Autodesk Inventor part; units mm, degrees
ref_plane "YZ Plane" through (0, 0, 0) normal (1, 0, 0) x (0, 1, 0)
ref_plane "XZ Plane" through (0, 0, 0) normal (0, 1, 0) x (-1, 0, 0)
ref_plane "XY Plane" through (0, 0, 0) normal (0, 0, 1) x (1, 0, 0)
sketch "Sketch1" plane through (0, 0, 0) normal (0, 0, 1) x (1, 0, 0)
  line L0 (0, 0) -> (10, 0)
  line L1 (10, 0) -> (10, 6)
  line L2 (10, 6) -> (0, 6)
  line L3 (0, 6) -> (0, 0)
  dimension "d0" = 10
  dimension "d1" = 6
extrude "Extrusion1" add sketch "Sketch1" along normal blind 4
sketch "Sketch2" plane through (0, 0, 4) normal (0, 0, 1) x (1, 0, 0)
  line L0 (1, 1) -> (9, 1)
  line L1 (9, 1) -> (9, 5)
  line L2 (9, 5) -> (1, 5)
  line L3 (1, 5) -> (1, 1)
  point P0 (0, 0)
  dimension "d4" = 8
  dimension "d5" = 4
extrude "Extrusion2" cut sketch "Sketch2" against normal blind 2.5
sketch "Sketch5" plane through (1, 1, 4) normal (0, 1, 0) x (1, 0, 0)
  circle A0 centre (1, 0.5) radius 0.25
  point P0 (-1, 4)
  dimension "d14" = 0.5
sketch "Sketch6" plane through (1, 1, 4) normal (0, 1, 0) x (1, 0, 0)
  circle A0 centre (7, 0.5) radius 0.25
  point P0 (-1, 4)
  dimension "d15" = 0.5
extrude "Extrusion4" add sketch "Sketch5" along normal blind 4
extrude "Extrusion5" add sketch "Sketch6" along normal blind 4
sketch "Sketch14" plane through (0, 0, 0) normal (0, 0, -1) x (-1, 0, 0)
  line L0 (0, 6) -> (0, 0)
  line L1 (0, 0) -> (-10, 0)
  line L2 (0, 6) -> (-10, 6)
  line L3 (-10, 6) -> (-10, 0)
  line L4 (-10, 0) -> (0, 0)
  line L5 (0, 0) -> (0, 6)
extrude "Extrusion12" add sketch "Sketch14" along normal blind 6
sketch "Sketch15" plane through (0, 0, 4) normal (-1, 0, 0) x (0, 0, 1)
  line L0 (-10, 0) -> (0, 0)
  line L1 (-10, 0) -> (-4, 0)
  line L2 (-4, 0) -> (-4, 6)
  line L3 (-4, 6) -> (-10, 6)
  line L4 (-10, 6) -> (-10, 0)
  point P0 (-4, 0)
  dimension "d42" = 6
  dimension "d43" = 6
extrude "Extrusion13" add sketch "Sketch15" along normal blind 5
sketch "Sketch16" plane through (-5, 0, 4) normal (-1, 0, 0) x (0, 0, 1)
  circle A0 centre (-7, 3) radius 2.25
  point P0 (-4, 0)
  dimension "d46" = 4.5
extrude "Extrusion14" cut sketch "Sketch16" against normal blind 15
sketch "Sketch17" plane through (0, 0, 1.5) normal (0, 0, 1) x (1, 0, 0)
  circle A0 centre (3, 3) radius 0.25
  point P0 (0, 0)
  dimension "d49" = 0.5
extrude "Extrusion15" add sketch "Sketch17" along normal blind 0.5
sketch "Sketch18" plane through (0, 0, 1.5) normal (0, 0, 1) x (1, 0, 0)
  circle A0 centre (5, 3) radius 0.25
  circle A1 centre (7, 3) radius 0.25
  circle A2 centre (4, 4) radius 0.25
  circle A3 centre (6, 4) radius 0.25
  circle A4 centre (4, 2) radius 0.25
  circle A5 centre (6, 2) radius 0.25
  point P0 (0, 0)
  dimension "d52" = 0.5
  dimension "d53" = 0.5
  dimension "d54" = 0.5
  dimension "d55" = 0.5
  dimension "d56" = 0.5
  dimension "d57" = 0.5
extrude "Extrusion16" add sketch "Sketch18" along normal blind 0.5
sketch "Sketch19" plane through (1, 1, 4) normal (0, 1, 0) x (1, 0, 0)
  point P0 (-1, 4)
sketch "Sketch20" plane through (1, 1, 4) normal (0, 1, 0) x (1, 0, 0)
  circle A0 centre (2, 1) radius 0.25
  circle A1 centre (4, 1) radius 0.25
  circle A2 centre (6, 1) radius 0.25
  point P0 (-1, 4)
  dimension "d60" = 0.5
  dimension "d61" = 0.5
  dimension "d62" = 0.5
extrude "Extrusion17" add sketch "Sketch20" along normal blind 0.8
sketch "Sketch21" plane through (1, 5, 4) normal (0, -1, 0) x (1, 0, 0)
  circle A0 centre (2, -1) radius 0.25
  circle A1 centre (4, -1) radius 0.25
  circle A2 centre (6, -1) radius 0.25
  point P0 (-1, -4)
  dimension "d65" = 0.5
  dimension "d66" = 0.5
  dimension "d67" = 0.5
extrude "Extrusion18" add sketch "Sketch21" along normal blind 0.8
sketch "Sketch22" plane through (0, 0, 0) normal (0, 0, 1) x (1, 0, 0)
  circle A0 centre (-2.5, 3) radius 1
  point P0 (0, 0)
  dimension "d70" = 2
extrude "Extrusion19" cut sketch "Sketch22" against normal blind 6
sketch "Sketch23" plane through (0, 0, 4) normal (0, -1, 0) x (1, 0, 0)
  point P0 (0, -4)
sketch "Sketch24" plane through (0, 0, 4) normal (0, -1, 0) x (1, 0, 0)
  circle A0 centre (-2.5, -7) radius 1
  point P0 (0, -4)
  dimension "d73" = 2
extrude "Extrusion20" cut sketch "Sketch24" against normal blind 6
properties part number "20190425_NewHolde3"
The listing builds one solid part. Answer for the finished solid, in the listing's coordinates (mm). A direction names the side the tool comes from. Coordinates: 2 decimals unless noted, no trailing zeros. Write each loop counter-clockwise with the first axis right and the second up, starting at its lowest first coordinate (ties: lowest second). Pieces come first, ordered by that corner, then holes.
Q1. Given P1, Ø0.6, axis at x = 4, y = 4, coming from the +Z side; P2, Ø3, axis at x = -2.5, y = 3, coming from the +Z side, each flat-ended and moving along its own axis, determine where each tip first touches the part or whether it passes through.
Returned:
P1: stops at z = 2
P2: stops at z = 0
Q2. The mould has two halves that part along Y. Classify faces 4 (the flat face through (10, 3, 0)), 5 (the flat face through (9, 3, 3)), 6 (the cylindrical face through (2.395, 3.099, -5.248)), 7 (the flat face through (4, 0, -1)): released by +Y, released by -Y, zero draft, split by the parting line, or undercut.
Returned:
face 4: zero draft
face 5: undercut
face 6: undercut
face 7: released by -Y
Q3. Find the intervals of material crossed by line 1 along X through (y, z) = (5.35, -3); line 2 along Y through (x, z) = (-2.5, -0.4); line 3 along X through (y, z) = (3.75, 2.5), in increasing order.
Returned:
line 1: x = -5 to -3.5, -1.5 to 10
line 2: y = 0 to 2, 4 to 6
line 3: x = 0 to 1, 9 to 10
Q4. Which of the six approach directions +Z, -Z, +X, -X, +Y, -Y give full straight-line access (tool end or side, diameter ignored) to faces 1 (the flat face through (1, 3, 3)), 2 (the flat face through (0, 3, 2)), 3 (the cylindrical face through (-3.3, 0.5, -3.6))?
Returned:
face 1: +Z
face 2: +Z, -X, +Y, -Y
face 3: +Y, -Y
Q5. Section B-B, the plane x = -1.75 is taken. Write down the section's boundary in (y, z).
Returned:
outline: (0, -6) - (2.34, -6) - (2.34, -5.15) arc R2.25 cw to (0.85, -3.66) - (0, -3.66) - close; (0, -2.34) - (0.85, -2.34) arc R2.25 cw to (2.34, -0.85) - (2.34, 0) - (0, 0) - close; (3.66, -6) - (6, -6) - (6, -3.66) - (5.15, -3.66) arc R2.25 cw to (3.66, -5.15) - close; (3.66, -0.85) arc R2.25 cw to (5.15, -2.34) - (6, -2.34) - (6, 0) - (3.66, 0) - close
Q6. Section D-D, the plane z = -0.5 is taken. Write down the section's boundary in (x, y).
Returned:
outline: (-5, 0) - (10, 0) - (10, 6) - (-5, 6) - close; hole circle Ø2 at (-2.5, 3)
Q7. Section A-A, the plane x = 3 is taken. Write down the section's boundary in (y, z), then the cut area to 3 significant figures.
Returned:
outline: (0, -6) - (6, -6) - (6, 4) - (5, 4) - (5, 3.25) - (4.2, 3.25) - (4.2, 2.75) - (5, 2.75) - (5, 1.5) - (3.25, 1.5) - (3.25, 2) - (2.75, 2) - (2.75, 1.5) - (1, 1.5) - (1, 2.75) - (1.8, 2.75) - (1.8, 3.25) - (1, 3.25) - (1, 4) - (0, 4) - close; hole circle Ø4.5 at (3, -3)
area: 35.1 mm2
Q8. Section C-C, the plane y = 5.5 is taken. Write down the section's boundary in (x, z), then the cut area to 3 significant figures.
Returned:
outline: (-5, -6) - (10, -6) - (10, 4) - (0, 4) - (0, 0) - (-5, 0) - close; hole circle Ø2 at (-2.5, -3)
area: 127 mm2
